Geometry check sheet. Reference: the model listing, model coordinates, mm. A direction names the side the tool comes from. Round coordinates to 2 decimals unless told otherwise and drop trailing zeros. Order: outer loops, then holes, each group sorted by start corner. A loop starts at its lowest first (then second) coordinate and runs counter-clockwise, first axis right, second up.
Autodesk Inventor part; units mm, degrees
ref_plane "YZ Plane" through (0, 0, 0) normal (1, 0, 0) x (0, 1, 0)
ref_plane "XZ Plane" through (0, 0, 0) normal (0, 1, 0) x (-1, 0, 0)
ref_plane "XY Plane" through (0, 0, 0) normal (0, 0, 1) x (1, 0, 0)
sketch "Sketch1" plane through (0, 0, 0) normal (0, 1, 0) x (-1, 0, 0)
  line L0 (-20.955, 20.955) -> (20.955, 20.955)
  line L1 (20.955, 20.955) -> (20.955, -20.955)
  line L2 (20.955, -20.955) -> (-20.955, -20.955)
  line L3 (-20.955, -20.955) -> (-20.955, 20.955)
  line L4 (-20.955, 20.955) -> (20.955, -20.955) construction
  line L5 (20.955, 20.955) -> (-20.955, -20.955) construction
  circle A0 centre (17.4625, -17.4625) radius 2.54
  circle A1 centre (-17.4625, 17.4625) radius 2.54
  line L6 (17.4625, -17.4625) -> (17.4625, 17.4625) construction
  line L7 (-17.4625, 17.4625) -> (-17.4625, -17.4625) construction
  line L8 (0, 20.955) -> (0, -20.955) construction
  point P0 (0, 0)
  dimension "d0" = 41.91
  dimension "d1" = 34.925
  dimension "d2" = 5.08
extrude "Extrusion1" add sketch "Sketch1" along normal blind 62.23
sketch "Sketch2" plane through (0, 0, 0) normal (0, -1, 0) x (1, 0, 0)
  circle A0 centre (0, 0) radius 19.812
  dimension "d5" = 39.624
extrude "Extrusion2" add sketch "Sketch2" along normal blind 71.12
sketch "Sketch3" plane through (0, -71.12, 0) normal (0, -1, 0) x (1, 0, 0)
  circle A0 centre (0, 0) radius 6.35
  dimension "d8" = 12.7
extrude "Extrusion3" add sketch "Sketch3" along normal blind 1.524
sketch "Sketch4" plane through (0, 62.23, 0) normal (0, 1, 0) x (1, 0, 0)
  circle A0 centre (0, 0) radius 6.35
  dimension "d11" = 12.7
extrude "Extrusion4" add sketch "Sketch4" along normal blind 40.64
sketch "Sketch5" plane through (20.955, 0, 20.955) normal (1, 0, 0) x (0, 0, -1)
  line L0 (8.255, 52.07) -> (33.655, 52.07) construction
  line L1 (33.655, 52.07) -> (33.655, 7.62) construction
  line L2 (33.655, 7.62) -> (8.255, 7.62) construction
  line L3 (8.255, 7.62) -> (8.255, 52.07) construction
  line L4 (20.955, 0) -> (20.955, 7.62) construction
  line L5 (0, 62.23) -> (41.91, 62.23) construction
  circle A0 centre (8.255, 52.07) radius 1.905
  circle A1 centre (33.655, 52.07) radius 1.905
  circle A2 centre (33.655, 7.62) radius 1.905
  circle A3 centre (8.255, 7.62) radius 1.905
  dimension "d14" = 25.4
  dimension "d15" = 44.45
  dimension "d16" = 10.16
  dimension "d17" = 3.81
extrude "Extrusion5" cut sketch "Sketch5" against normal through all
properties part number "micro cim"
(1) Sectioned sample at C-C, the plane y = 52.07. Record the cut outline in (x, z) (1 decimal), and give its area (3 significant figures).
Returned:
outline: (-21, -21) - (21, -21) - (21, -14.6) - (-21, -14.6) - close; (-21, -10.8) - (21, -10.8) - (21, 10.8) - (-21, 10.8) - close; (-21, 14.6) - (21, 14.6) - (21, 21) - (-21, 21) - close; hole circle Ø5.1 at (-17.5, -17.5); hole circle Ø5.1 at (17.5, 17.5)
area: 1,400 mm2
(2) Sectioned sample at B-B, the plane z = 0. Record the cut outline in (x, y) (3 decimals).
Returned:
outline: (-20.955, 0) - (-19.812, 0) - (-19.812, -71.12) - (-6.35, -71.12) - (-6.35, -72.644) - (6.35, -72.644) - (6.35, -71.12) - (19.812, -71.12) - (19.812, 0) - (20.955, 0) - (20.955, 62.23) - (6.35, 62.23) - (6.35, 102.87) - (-6.35, 102.87) - (-6.35, 62.23) - (-20.955, 62.23) - close
(3) Depth check by flat-ended pin: P1, Ø5, axis at x = -14.5, z = 5.5, coming from the -Y side; P2, Ø2.5, axis at y = 52.07, z = -12.7, coming from the +X side; P3, Ø12, axis at y = -41.5, z = -5.5, coming from the -X side; P4, Ø12, axis at x = -14, z = -3, coming from the +Y side. Enter the tip coordinate at first touch or a pass-through.
Returned:
P1: stops at y = -71.12
P2: passes through
P3: stops at x = -19.81
P4: stops at y = 62.23
(4) Set-up check for faces 4 (the flat face through (5, 62.23, 5)), 5 (the cylindrical face through (-2.579, -35.062, -19.643)), 6 (the cylindrical face through (0.293, 8.192, -14.517)): record each of +Z, -Z, +X, -X, +Y, -Y from which the full face is reachable in a straight line by a thin tool's end or side.
Returned:
face 4: +Y
face 5: -Y
face 6: +X, -X
(5) Sectioned sample at D-D, the plane y = 25. Record the cut outline in (x, z) (1 decimal).
Returned:
outline: (-21, -21) - (21, -21) - (21, 21) - (-21, 21) - close; hole circle Ø5.1 at (-17.5, -17.5); hole circle Ø5.1 at (17.5, 17.5)
(6) Sectioned sample at A-A, the plane x = 0. Record the cut outline in (y, z) (3 decimals), and give its area (3 significant figures).
Returned:
outline: (-72.644, -6.35) - (-71.12, -6.35) - (-71.12, -19.812) - (0, -19.812) - (0, -20.955) - (62.23, -20.955) - (62.23, -6.35) - (102.87, -6.35) - (102.87, 6.35) - (62.23, 6.35) - (62.23, 20.955) - (0, 20.955) - (0, 19.812) - (-71.12, 19.812) - (-71.12, 6.35) - (-72.644, 6.35) - close; hole circle Ø3.81 at (7.62, -12.7); hole circle Ø3.81 at (7.62, 12.7); hole circle Ø3.81 at (52.07, -12.7); hole circle Ø3.81 at (52.07, 12.7)
area: 5,920 mm2
(7) Draft check along Z on faces 1 (the flat face through (-5, -71.12, 5)), 2 (the cylindrical face through (0.293, 7.704, 14.603)), 3 (the cylindrical face through (-1.38, 82.27, -6.2)). Enter one of: released by +Z, released by -Z, zero draft, split by the parting line, or undercut.
Returned:
face 1: zero draft
face 2: undercut
face 3: split by the parting line
(8) Material ranges on line 1 (Y direction, x = -1, z = -12.5); line 2 (Y direction, x = 0, z = -12); line 3 (Y direction, x = 8, z = 5.5), recorded low to high.
Returned:
line 1: y = -71.12 to 5.73, 9.51 to 50.18, 53.96 to 62.23
line 2: y = -71.12 to 5.85, 9.39 to 50.3, 53.84 to 62.23
line 3: y = -71.12 to 62.23
